Job drawing, mm, ordinate dimensions from the low corner. One solid piece. Give positions to 0.01 mm unless a question says otherwise; leave off trailing zeros. Loops run counter-clockwise (first coordinate to the right, second up) from the corner with the lowest first, then second, coordinate; pieces in that order, holes last. Notation, with made-up numbers: (-6.75, 60.5) - (16.25, 60.5) arc R14 ccw to (16.25, 72.5) - close; hole circle Ø9 at (25, 50.25). An arc over 180 degrees is marked (long way). Answer as CSV lines item,"result". Start each with the question number.
Item 1: Pull direction Y, two halves, no side cores. Call the marked faces 1, 2 and 3: pulls with the +Y half, pulls with the -Y half, needs draft (parallel to the pull), parting line crosses it, or undercut.
Item 2: Saw through at C-C on z = 0.55. Give the cut face in (x, y).
Item 3: Drill centre lines: L1, parallel to Z at x = 5, y = 11; L2, parallel to Y at x = 1.75, z = 0.85 (1 decimal); L3, parallel to Y at x = 9, z = 1.25 (1 decimal). Where is each one in solid material? Low to high. Write a range as from..to.
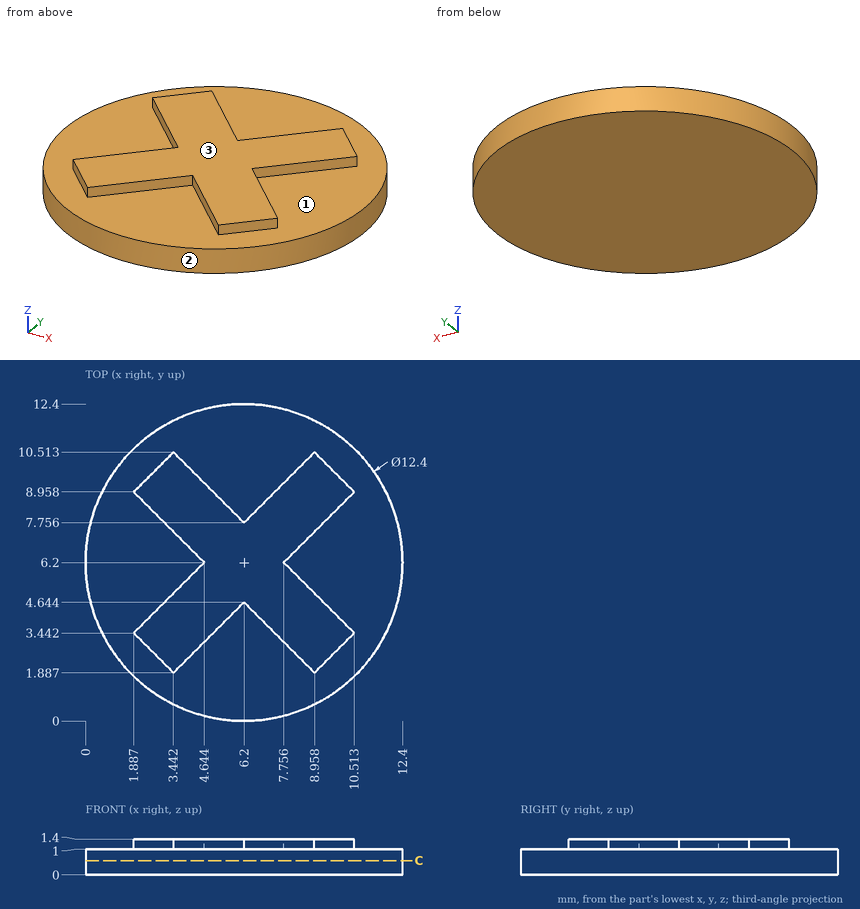
Responses:
1,face 1,"undercut"
1,face 2,"parting line crosses it"
1,face 3,"needs draft"
2,outline,"circle Ø12.4 at (6.2, 6.2)"
3,L1,"0..1"
3,L2,"1.9..10.5"
3,L3,"1.9..5, 7.4..10.5"
